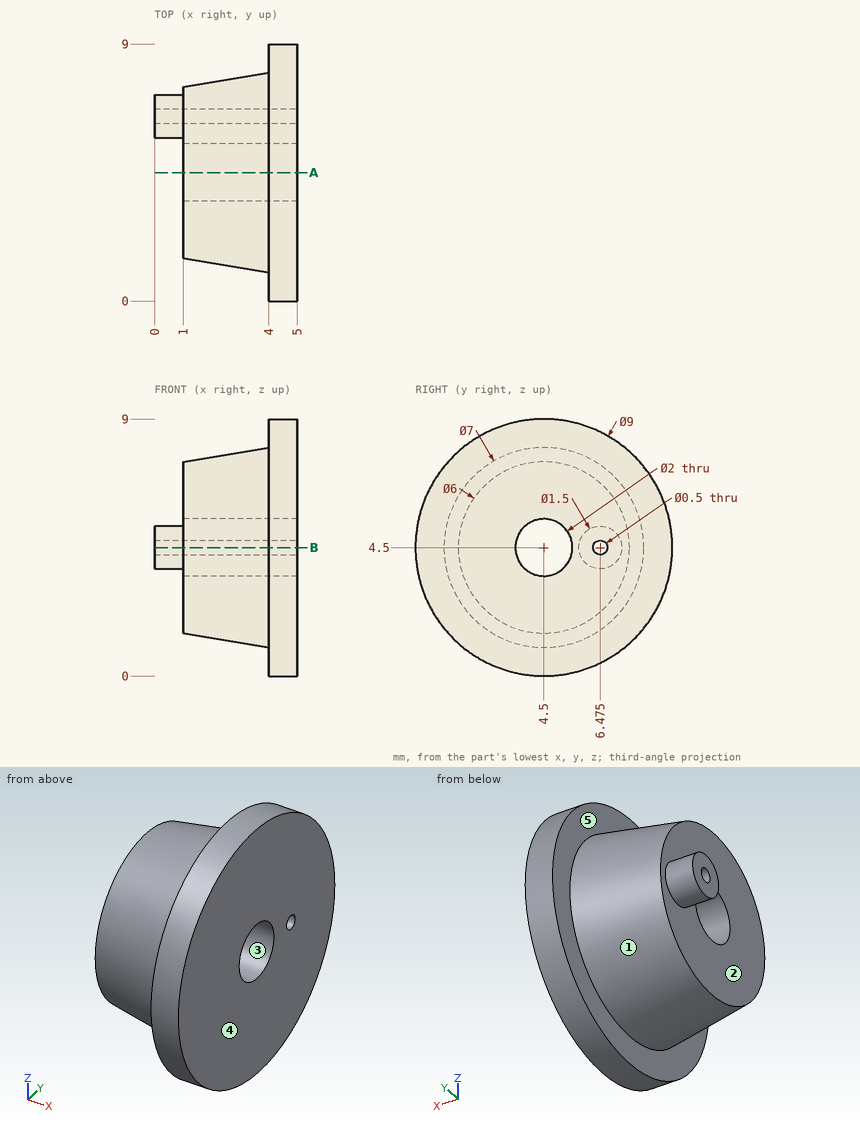
The figure shows three views and two pictorial views of one solid part (mm, origin at its lowest corner). Answer the questions. A direction names the side the tool comes from. Give positions to 0.01 mm unless a question says otherwise; leave off trailing zeros. Write each loop counter-clockwise with the first axis right and the second up, starting at its lowest first coordinate (ties: lowest second). Pieces come first, ordered by that corner, then holes. Notation, with made-up numbers: (17, 42) -> (42, 42) arc R16 ccw to (42, 55) -> close; hole circle Ø5 at (10.5, 78). An arc over 180 degrees is marked (long way). Write each question's results on one line, items separated by ' | '.
1. Determine the mould class of the marked faces 1, 2 and 3 for opening direction Z: +Z half, -Z half, draft (parallel to the pull), parting line (faces both ways), or undercut.
Data:
face 1: parting line | face 2: draft | face 3: undercut
2. This flat-tipped pin is pushed along its axis until it touches: pin 1 Ø4 at (y, z) = (1.5, 5) entering from -X. Where does it stop, or does it pass through?
Data:
pin 1: x = 1
3. A tool of negligible diameter and unlimited length cuts with its end or side. For the marked faces 4 and 5, from which of +Z, -Z, +X, -X, +Y, -Y can it reach the whole face along a straight path? Write none if from no direction.
Data:
face 4: +Z, -Z, +X, +Y, -Y | face 5: -X
4. Find section A-A on y = 4.5. Determine the outline of the cut face in (x, z), and give its area (3 significant figures).
Data:
outline: (1, 1.5) -> (4, 1) -> (4, 0) -> (5, 0) -> (5, 3.5) -> (1, 3.5) -> close; (1, 5.5) -> (5, 5.5) -> (5, 9) -> (4, 9) -> (4, 8) -> (1, 7.5) -> close | area: 20.5 mm^2
5. Find section B-B on z = 4.5. Give the number of separate pieces and of enclosed holes in the cut face, and give its area (3 significant figures).
Data:
separate pieces: 3 | enclosed holes: 0 | area: 19.5 mm^2
6. Straight lines are drawn through the part: L1, parallel to Z at x = 4.1, y = 4.5; L2, parallel to X at y = 5, z = 6.5; L3, parallel to Z at x = 2.7, y = 4.5. For each, find the intervals that lie inside material, in ascending order.
Data:
L1: 0 to 3.5, 5.5 to 9 | L2: 1 to 5 | L3: 1.22 to 3.5, 5.5 to 7.78
